```python
from build123d import *

# Parameters (mm, degrees)
EXTRUDE_1_DEPTH     = 50
SKETCH_4_R          = 20
CUT_EXTRUDE_1_DEPTH = 96.654466254
SKETCH_6_R          = 115.5
CUT_EXTRUDE_3_DEPTH = 20
SKETCH_8_R          = 2.75
CUT_EXTRUDE_4_DEPTH = 10
FILLET_1_R          = 3


with BuildPart() as part:
    # Sketch 1 → Extrude 1 (new body)
    with BuildSketch(Plane.XY):
        Polygon((-24.51528993, 0), (0, 0), (69.48471007, -8.477916399), (69.48471007, 0.522083601), (-0.51528993, 26), (-24.51528993, 26), align=None)
    extrude(amount=EXTRUDE_1_DEPTH)

    # Sketch 4 → Cut-Extrude 1 (cut, through all)
    with BuildSketch(Plane(origin=(-8.811251384, 3.207033231, 0), x_dir=(0, 0, 1), z_dir=(-0.9396926207859082, 0.34202014332566955, 0))):
        with Locations((25, 36.255768605)):
            Circle(SKETCH_4_R)
    extrude(amount=-CUT_EXTRUDE_1_DEPTH, mode=Mode.SUBTRACT)

    # Sketch 6 → Cut-Extrude 3 (cut)
    with BuildSketch(Plane(origin=(0, 26, 0), x_dir=(1, 0, 0), z_dir=(0, 1, 0))):
        with Locations((-112.01528993, -25)):
            Circle(SKETCH_6_R)
    extrude(amount=-CUT_EXTRUDE_3_DEPTH, mode=Mode.SUBTRACT)

    # Sketch 8 → Cut-Extrude 4 (cut)
    with BuildSketch(Plane.XZ):
        with Locations(Location((-8, 40, 0), (0, 0, 270))):
            Circle(SKETCH_8_R)
        with Locations(Location((-8, 10, 0), (0, 0, 180))):
            Circle(SKETCH_8_R)
    extrude(amount=-CUT_EXTRUDE_4_DEPTH, mode=Mode.SUBTRACT)

    # Fillet 1
    fillet_1_edges = [part.edges().sort_by_distance(p)[0] for p in [
        (3.48471007, 16.030696883, 25),
    ]]
    fillet(fillet_1_edges, radius=FILLET_1_R)


solid = part.part
```
Here's how the part is built. I have some questions about the finished solid (model axes, mm). A direction names the side the tool comes from. Coordinates: 2 decimals unless noted, no trailing zeros. Order: outer loops, then holes, each group sorted by start corner. A loop starts at its lowest first (then second) coordinate and runs counter-clockwise, first axis right, second up.
1) We'd pull the mould along Z, two halves only. Please class faces 4 (the face through (22, 5, 50)), 5 (the face through (-10.62, 2.96, 9.17)), 6 (the face through (35.597, 12.856, 45.437)): +Z half, -Z half, draft (parallel to the pull), parting line (faces both ways), or undercut.
2) Imagine slicing it at A-A on x = -8. List the corners of the cut face in (y, z) for me, and give its area (3 significant figures).
3) I need wall thicknesses on line 1 (Y direction, x = -6, z = 26); line 2 (Z direction, x = 23.5, y = 12.5); line 3 (Z direction, x = 61.5, y = 2). Which ranges of each line are inside material? Lowest first, please.
4) Which directions (+Z, -Z, +X, -X, +Y, -Y) give clear straight access to the entire face, cutting with the end or side of a thin tool? Please do faces 1 (the face through (35.597, 12.856, 4.437)), 2 (the face through (3.484, 11.565, 25.353)), 3 (the face through (-12, 0, 25)).
5) Will these pins go through, and if not, where does the flat tip stop? pin 1 (3.5 mm diameter, centred on x = -8, z = 40, fed in from -Y); pin 2 (7 mm diameter, centred on x = -8, z = 10, fed in from -Y); pin 3 (2 mm diameter, centred on x = 1, z = 24, fed in from -Y); pin 4 (1.5 mm diameter, centred on x = 59.5, z = 19, fed in from -Y).
Response values:
1. face 4: +Z half
1. face 5: undercut
1. face 6: draft
2. outline: (0, 0) - (6, 0) - (6, 7.25) - (0, 7.25) - close; (0, 12.75) - (6, 12.75) - (6, 37.25) - (0, 37.25) - close; (0, 42.75) - (6, 42.75) - (6, 50) - (0, 50) - close
2. area: 234 mm2
3. line 1: y = 0 to 6
3. line 2: z = 0 to 13.66, 36.34 to 50
3. line 3: z = 0 to 10.1, 39.9 to 50
4. face 1: +Z, -Z, +X, +Y
4. face 2: -X, +Y
4. face 3: +Z, -Z, -X, -Y
5. pin 1: passes through
5. pin 2: stops at y = 0
5. pin 3: stops at y = -0.24
5. pin 4: stops at y = -7.35
